from build123d import *

# Parameters (mm, degrees)
SKETCH_1_R                   = 10
EXTRUDE_1_DEPTH              = 4
SKETCH_4_R                   = 1.65
CUT_EXTRUDE_1_DEPTH          = 4
SKETCH_5_R                   = 5
EXTRUDE_2_DEPTH              = 11
HOLE_WIZARD_M8_1_D           = 6.8
HOLE_WIZARD_M8_1_ON_FACE_2_D = 6.8
CUT_EXTRUDE_4_DEPTH          = 24.450776575
CUT_EXTRUDE_4_DEPTH_BACK     = 24.450776575
SKETCH_11_W                  = 3.417857142
SKETCH_11_H                  = 2.9
SKETCH_12_R                  = 4.6
CUT_EXTRUDE_5_DEPTH          = 2.85


with BuildPart() as part:
    # 草图1 → 凸台-拉伸1 (new body)
    with BuildSketch(Plane(origin=(0, 0, 0), x_dir=(1, 0, 0), z_dir=(0, 1, 0))):
        with Locations(Location((0, 0, 0), (0, 0, 270))):
            Circle(SKETCH_1_R)
    extrude(amount=EXTRUDE_1_DEPTH)

    # 草图4 → 切除-拉伸1 (cut)
    with BuildSketch(Plane(origin=(0, 0, 0), x_dir=(-1, 0, 0), z_dir=(0, -1, 0))):
        with Locations(Location((5.400107697, -5.902443296, 0), (0, 0, 90))):
            Circle(SKETCH_4_R)
        with Locations(Location((-5.400107697, -5.902443296, 0), (0, 0, 90))):
            Circle(SKETCH_4_R)
        with Locations(Location((-5.400107697, 5.902443296, 0), (0, 0, 90))):
            Circle(SKETCH_4_R)
        with Locations(Location((5.400107697, 5.902443296, 0), (0, 0, 90))):
            Circle(SKETCH_4_R)
    extrude(amount=-CUT_EXTRUDE_1_DEPTH, mode=Mode.SUBTRACT)

    # 草图5 → 凸台-拉伸2 (add)
    with BuildSketch(Plane(origin=(0, 4, 0), x_dir=(1, 0, 0), z_dir=(0, 1, 0))):
        with Locations(Location((0, 0, 0), (0, 0, 270))):
            Circle(SKETCH_5_R)
    extrude(amount=EXTRUDE_2_DEPTH)

    # M8 螺纹孔1 (through all)
    with Locations(Plane(origin=(0, 0, 0), x_dir=(0, 0, -1), z_dir=(0, -1, 0))):
        with Locations((0, 0)):
            Hole(HOLE_WIZARD_M8_1_D / 2)

    # M8 螺纹孔1 on face 2 (through all)
    with Locations(Plane.ZX.offset(15)):
        with Locations((0, 0)):
            Hole(HOLE_WIZARD_M8_1_ON_FACE_2_D / 2)

    # 草图11 → 切除-拉伸4 (cut, two sides: drawn at the far end of the back side and taken through both)
    with BuildSketch(Plane(origin=(4.997963928, 0, 0), x_dir=(0, 0, -1), z_dir=(1, 0, 0)).offset(-CUT_EXTRUDE_4_DEPTH_BACK)):
        with Locations((0, 13.597531036)):
            Rectangle(SKETCH_11_W, SKETCH_11_H)
    extrude(amount=CUT_EXTRUDE_4_DEPTH + CUT_EXTRUDE_4_DEPTH_BACK, mode=Mode.SUBTRACT)

    # 草图12 → 切除-拉伸5 (cut)
    with BuildSketch(Plane(origin=(0, 15, 0), x_dir=(1, 0, 0), z_dir=(0, 1, 0))):
        Circle(SKETCH_12_R)
    extrude(amount=-CUT_EXTRUDE_5_DEPTH, mode=Mode.SUBTRACT)


solid = part.part
Read the model definition and answer for the solid it produces. Units are mm, in the model's axes. A direction names the side the tool comes from. Round coordinates to 2 decimals unless told otherwise and drop trailing zeros. Write each loop counter-clockwise with the first axis right and the second up, starting at its lowest first coordinate (ties: lowest second). Pieces come first, ordered by that corner, then holes. Notation, with made-up numbers: M 48,43 L 75,43 A15 cw 75,63 Z; hole C 23.5,61.5 d5. An arc over 180 degrees is marked long. Use a Markdown table: item, result.
1) The part is cut by section A-A (x = 0). Write down the section's boundary in (y, z).
Answers follow:
| item | result |
|---|---|
| outline | M 0,-10 L 4,-10 L 4,-5 L 15,-5 L 15,-4.6 L 12.15,-4.6 L 12.15,-3.4 L 0,-3.4 Z; M 0,3.4 L 12.15,3.4 L 12.15,4.6 L 15,4.6 L 15,5 L 4,5 L 4,10 L 0,10 Z |
2) A tool of negligible diameter and unlimited length cuts with its end or side. For faces 1 (the flat face through (0, 12.15, -4)), 2 (the cylindrical face through (-6.404, 1.972, 7.212)), 3 (the flat face through (-4.5, 13.6, 1.709)), from which of +Z, -Z, +X, -X, +Y, -Y can it reach the whole face along a straight path? Write none if from no direction.
Answers follow:
| item | result |
|---|---|
| face 1 | +Y |
| face 2 | +Y, -Y |
| face 3 | +X, -X, +Y |
3) The part is cut by section D-D (y = 2). Write down the section's boundary in (x, z), plus the area to 3 significant figures.
Answers follow:
| item | result |
|---|---|
| outline | C 0,0 d20; hole C -5.4,-5.9 d3.3; hole C -5.4,5.9 d3.3; hole C 0,0 d6.8; hole C 5.4,-5.9 d3.3; hole C 5.4,5.9 d3.3 |
| area | 244 mm2 |
4) The part is cut by section B-B (z = 0). Write down the section's boundary in (x, y), plus the area to 3 significant figures.
Answers follow:
| item | result |
|---|---|
| outline | M -10,0 L -3.4,0 L -3.4,12.15 L -5,12.15 L -5,4 L -10,4 Z; M 3.4,0 L 10,0 L 10,4 L 5,4 L 5,12.15 L 3.4,12.15 Z |
| area | 78.9 mm2 |
5) Flat-ended cylindrical pins translate along their axes: pin 1 (1.4 mm diameter, centred on x = -3.5, y = 13, fed in from -Z); pin 2 (0.9 mm diameter, centred on x = -3.5, y = 14, fed in from +Z); pin 3 (3 mm diameter, centred on y = 8.5, z = -3.5, fed in from +X). Find the tip coordinate at first contact, or state that the pin passes through.
Answers follow:
| item | result |
|---|---|
| pin 1 | stops at z = -4.14 |
| pin 2 | stops at z = 3.96 |
| pin 3 | stops at x = 4.58 |
6) Straight lines are drawn through the part: line 1 along Z through (x, y) = (0.25, 13); line 2 along Z through (x, y) = (-5, 1.75); line 3 along Y through (x, z) = (3.25, -7.75). For each, find the intervals that lie inside material, in ascending order. Write a range as [from, to].
Answers follow:
| item | result |
|---|---|
| line 1 | z = [-4.99, -4.59], [4.59, 4.99] |
| line 2 | z = [-8.66, -7.5], [-4.3, 4.3], [7.5, 8.66] |
| line 3 | y = [0, 4] |
7) The part is cut by section C-C (z = -6). Write down the section's boundary in (x, y).
Answers follow:
| item | result |
|---|---|
| outline | M -8,0 L -7.05,0 L -7.05,4 L -8,4 Z; M -3.75,0 L 3.75,0 L 3.75,4 L -3.75,4 Z; M 7.05,0 L 8,0 L 8,4 L 7.05,4 Z |
8) For a pull along X with two mould halves and no side action, classify faces 4 (the cylindrical face through (-0.1, 13.6, 4.6)), 5 (the flat face through (0, 0, 4)), 6 (the cylindrical face through (4.396, 1.972, 7.212)), 7 (the cylindrical face through (-9.76, 1.97, -2.17)) as pulls with the +X half, pulls with the -X half, needs draft (parallel to the pull), parting line crosses it, or undercut.
Answers follow:
| item | result |
|---|---|
| face 4 | undercut |
| face 5 | needs draft |
| face 6 | undercut |
| face 7 | parting line crosses it |
